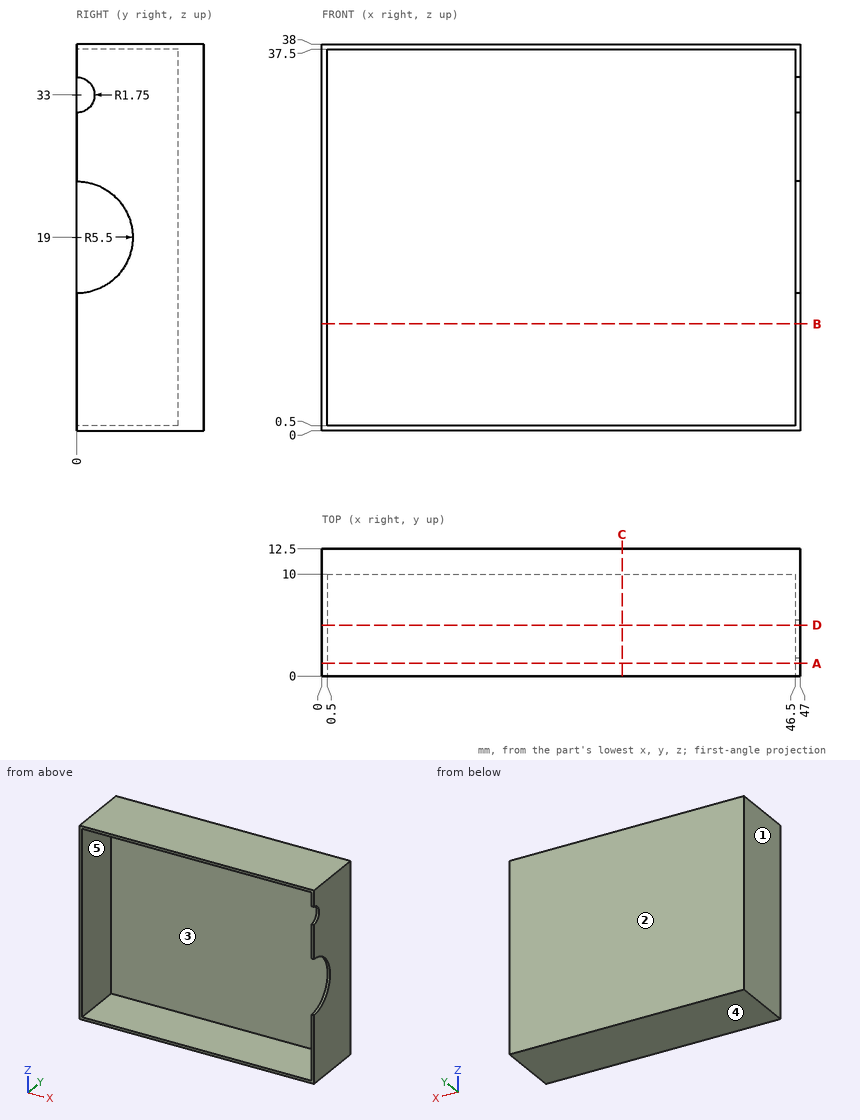
Source: three-view drawing plus pictorial views. Frame: mm from the lowest corner of the part. A direction names the side the tool comes from. Give positions to 0.01 mm unless a question says otherwise; leave off trailing zeros. Order: outer loops, then holes, each group sorted by start corner. A loop starts at its lowest first (then second) coordinate and runs counter-clockwise, first axis right, second up. Notation, with made-up numbers: M 33.5,31.5 L 82.5,31.5 A25 cw 82.5,63.5 Z; hole C 26,84.5 d7. An arc over 180 degrees is marked long. One line per question, with ' | ' between items. Start each with the question number.
1. Material intervals for probe 1 along Z at (x, y) = (32.5, 5.75); probe 2 along X at (y, z) = (5, 30); probe 3 along Y at (x, z) = (3, 4), sorted ascending. Write a range as [from, to].
2. Section query D-D (y = 5). Return the cut outline in (x, z).
3. Pull-direction query (X, two-part tool) for the marked faces 1, 2 and 3; classes: released by +X, released by -X, zero draft, split by the parting line, or undercut.
4. Section query A-A (y = 1.25). Return the cut outline in (x, z).
5. First-contact query: pin 1 Ø5 at (y, z) = (2.5, 16.5) entering from -X; pin 2 Ø2 at (x, z) = (33, 31) entering from -Y. Flat tips, straight axial feed; report the tip coordinate or a pass-through.
6. Section query B-B (z = 10.5). Return the cut outline in (x, y).
7. Access query for the marked faces 4 and 5. Directions: +Z, -Z, +X, -X, +Y, -Y. A direction counts if a zero-diameter tool reaches every point of the face in a straight line with its end or side. Return the directions, or none.
8. Section query C-C (x = 29.5). Return the cut outline in (y, z), and give its area (3 significant figures).
Here are the results:
1) probe 1: [0, 0.5], [37.5, 38] | probe 2: [0, 0.5], [46.5, 47] | probe 3: [10, 12.5]
2) outline: M 0,0 L 47,0 L 47,16.71 L 46.5,16.71 L 46.5,0.5 L 0.5,0.5 L 0.5,37.5 L 46.5,37.5 L 46.5,21.29 L 47,21.29 L 47,38 L 0,38 Z
3) face 1: released by -X | face 2: zero draft | face 3: undercut
4) outline: M 0,0 L 47,0 L 47,13.64 L 46.5,13.64 L 46.5,0.5 L 0.5,0.5 L 0.5,37.5 L 46.5,37.5 L 46.5,34.22 L 47,34.22 L 47,38 L 0,38 Z; M 46.5,24.36 L 47,24.36 L 47,31.78 L 46.5,31.78 Z
5) pin 1: x = 0 | pin 2: y = 10
6) outline: M 0,0 L 0.5,0 L 0.5,10 L 46.5,10 L 46.5,0 L 47,0 L 47,12.5 L 0,12.5 Z
7) face 4: -Z, +X, -X, +Y, -Y | face 5: -Y
8) outline: M 0,0 L 12.5,0 L 12.5,38 L 0,38 L 0,37.5 L 10,37.5 L 10,0.5 L 0,0.5 Z | area: 105 mm²
